Here's the drawing with two shaded views (mm, measured from the low corner). I have some questions. Coordinates: 2 decimals unless noted, no trailing zeros. Order: outer loops, then holes, each group sorted by start corner. A loop starts at its lowest first (then second) coordinate and runs counter-clockwise, first axis right, second up. Notation, with made-up numbers: (-16, -3) -> (39, -3) arc R35 ccw to (39, 35) -> close; hole circle Ø10 at (78.25, -19). An arc over 180 degrees is marked (long way). One line per item, written item: value. Start each with the question number.
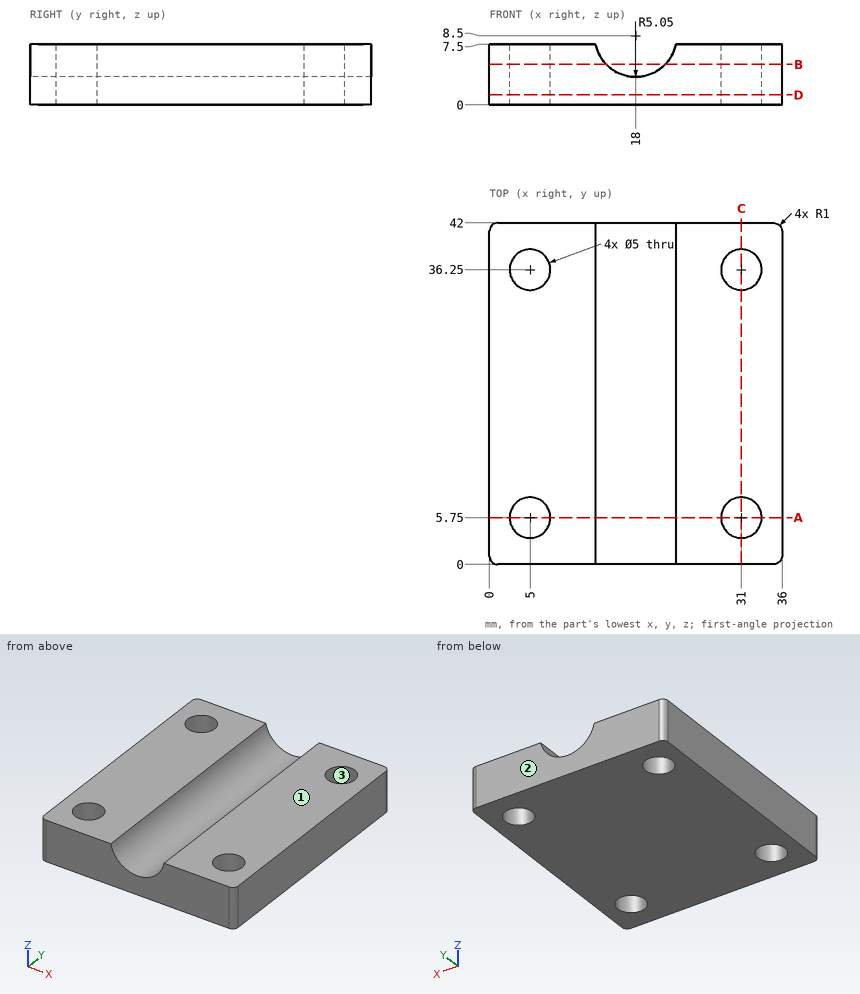
Q1. Imagine slicing it at B-B (z = 5). Write out the boundary of the cut face in (x, y), plus the area to 3 significant figures.
Q2. If we mould it in two halves opening along Y, with no side actions, what happens to the marked faces 1, 2 and 3? For each: +Y half, -Y half, draft (parallel to the pull), parting line (faces both ways), or undercut.
Q3. I need wall thicknesses on line 1 (Y direction, x = 5, z = 5.5); line 2 (X direction, y = 36.25, z = 3.25); line 3 (X direction, y = 36.25, z = 5.5). Which ranges of each line are inside material? Lowest first, please.
Q4. Imagine slicing it at C-C (x = 31). Write out the boundary of the cut face in (y, z), plus the area to 3 significant figures.
Q5. Imagine slicing it at D-D (z = 1.25). Write out the boundary of the cut face in (x, y).
Q6. Imagine slicing it at A-A (y = 5.75). Write out the boundary of the cut face in (x, z), plus the area to 3 significant figures.
Q7. For P1, Ø4, axis at x = 5, y = 5.75, coming from the -Z side, with a flat end and sliding along its axis, tell me the tip position at first contact or that it passes through.
Completed:
1. outline: (0, 1) arc R1 ccw to (1, 0) -> (14.36, 0) -> (14.36, 42) -> (1, 42) arc R1 ccw to (0, 41) -> close; (21.64, 0) -> (35, 0) arc R1 ccw to (36, 1) -> (36, 41) arc R1 ccw to (35, 42) -> (21.64, 42) -> close; hole circle Ø5 at (5, 5.75); hole circle Ø5 at (5, 36.25); hole circle Ø5 at (31, 5.75); hole circle Ø5 at (31, 36.25)
1. area: 1,130 mm2
2. face 1: draft
2. face 2: +Y half
2. face 3: undercut
3. line 1: y = 0 to 3.25, 8.25 to 33.75, 38.75 to 42
3. line 2: x = 0 to 2.5, 7.5 to 28.5, 33.5 to 36
3. line 3: x = 0 to 2.5, 7.5 to 13.94, 22.06 to 28.5, 33.5 to 36
4. outline: (0, 0) -> (3.25, 0) -> (3.25, 7.5) -> (0, 7.5) -> close; (8.25, 0) -> (33.75, 0) -> (33.75, 7.5) -> (8.25, 7.5) -> close; (38.75, 0) -> (42, 0) -> (42, 7.5) -> (38.75, 7.5) -> close
4. area: 240 mm2
5. outline: (0, 1) arc R1 ccw to (1, 0) -> (35, 0) arc R1 ccw to (36, 1) -> (36, 41) arc R1 ccw to (35, 42) -> (1, 42) arc R1 ccw to (0, 41) -> close; hole circle Ø5 at (5, 5.75); hole circle Ø5 at (5, 36.25); hole circle Ø5 at (31, 5.75); hole circle Ø5 at (31, 36.25)
6. outline: (0, 0) -> (2.5, 0) -> (2.5, 7.5) -> (0, 7.5) -> close; (7.5, 0) -> (28.5, 0) -> (28.5, 7.5) -> (22.95, 7.5) arc R5.05 cw to (13.05, 7.5) -> (7.5, 7.5) -> close; (33.5, 0) -> (36, 0) -> (36, 7.5) -> (33.5, 7.5) -> close
6. area: 165 mm2
7. P1: passes through
